Part model, mm, in its own coordinate system. Face numbers are marked on the shaded views. A direction names the side the tool comes from. Coordinates: 2 decimals unless noted, no trailing zeros. Write each loop counter-clockwise with the first axis right and the second up, starting at its lowest first coordinate (ties: lowest second). Pieces come first, ordered by that corner, then holes. Notation, with made-up numbers: M -19.5,23.25 L -15.5,23.25 A31 ccw -15.5,61.25 Z; hole C 87,43.25 d11. An arc over 180 degrees is marked long. Use a Markdown table: item, result. Add a question column.
Q1. Mould opens along Z. For the marked faces 1, 2 and 3 say: released by +Z, released by -Z, zero draft, split by the parting line, or undercut.
Q2. Pin check, flat tips, straight feed: pin 1 Ø3 at (x, y) = (9.5, 1) entering from +Z; pin 2 Ø0.9 at (x, y) = (1, 0) entering from -Z (3 decimals); pin 3 Ø3 at (x, z) = (6.5, -2.5) entering from +Y; pin 4 Ø4 at (x, z) = (2, -2.5) entering from -Y. Stop position of each tip, or through.
Q3. Slice it at B-B on x = 4. Write the cut outline in (y, z), then the cut area to 3 significant figures.
Q4. Tool access for the marked faces 4, 5 and 6: list every direction of +Z, -Z, +X, -X, +Y, -Y with a clear straight run to the whole face (end or side of a thin tool).
Q5. Slice it at A-A on x = 1.75. Write the cut outline in (y, z).
Q6. Wall check: L1, parallel to Z at x = 1.75, y = -0.5; L2, parallel to Y at x = 7, z = -1; L3, parallel to Y at x = 5, z = -2. Give the ranges that are in metal, low to high. Write a range as from..to.
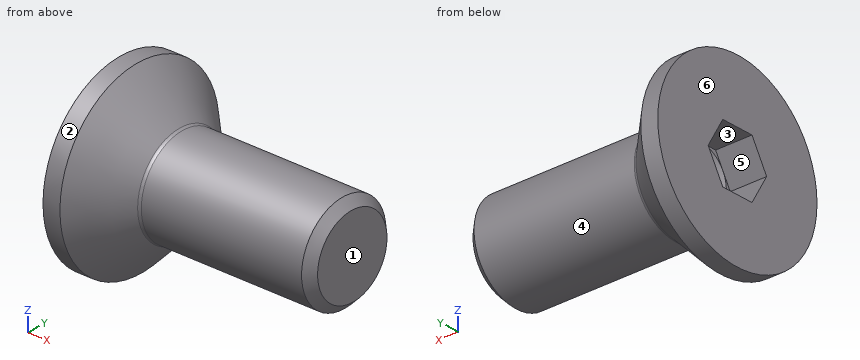
from build123d import *

# Parameters (mm, degrees)
FILLET1_R   = 0.2
HEX_2_DEPTH = 1.9


with BuildPart() as part:
    # BodySke → BaseBody (revolve)
    with BuildSketch(Plane.XY):
        Polygon((0, 0), (0, 4.715), (0.885, 4.715), (3.1, 2.5), (11.555, 2.5), (12, 2.055), (12, 0), align=None)
    revolve(axis=Axis((0, 0, 0), (1, 0, 0)))

    # Fillet1
    fillet1_edges = [part.edges().sort_by_distance(p)[0] for p in [
        (3.1, -2.5, 0),
    ]]
    fillet(fillet1_edges, radius=FILLET1_R)

    # Sketch2 → PreBroach (revolve, cut)
    with BuildSketch(Plane.XY):
        Polygon((0, 1.5), (1.9, 1.5), (2.766025404, 0), (0, 0), align=None)
    revolve(axis=Axis((0, 0, 0), (1, 0, 0)), mode=Mode.SUBTRACT)

    # Sketch3 → Hex 2 (cut)
    with BuildSketch(Plane.ZY):
        Polygon((-1.5, -0.866025404), (-1.5, 0.866025404), (0, 1.732050808), (1.5, 0.866025404), (1.5, -0.866025404), (0, -1.732050808), align=None)
    extrude(amount=-HEX_2_DEPTH, mode=Mode.SUBTRACT)


solid = part.part
Recorded:
| question | item | result |
|---|---|---|
| 1 | face 1 | zero draft |
| 1 | face 2 | split by the parting line |
| 1 | face 3 | undercut |
| 2 | pin 1 | z = 2.5 |
| 2 | pin 2 | z = -4.715 |
| 2 | pin 3 | y = 2.29 |
| 2 | pin 4 | y = -4.64 |
| 3 | outline | C 0,0 d5 |
| 3 | area | 19.6 mm² |
| 4 | face 4 | +X |
| 4 | face 5 | -X |
| 4 | face 6 | +Z, -Z, -X, +Y, -Y |
| 5 | outline | C 0,0 d7.7; hole M -1.73,0 L -0.87,-1.5 L 0.87,-1.5 L 1.73,0 L 0.87,1.5 L -0.87,1.5 Z |
| 6 | L1 | -3.82..-1.5, 1.5..3.82 |
| 6 | L2 | -2.29..2.29 |
| 6 | L3 | -1.5..1.5 |
